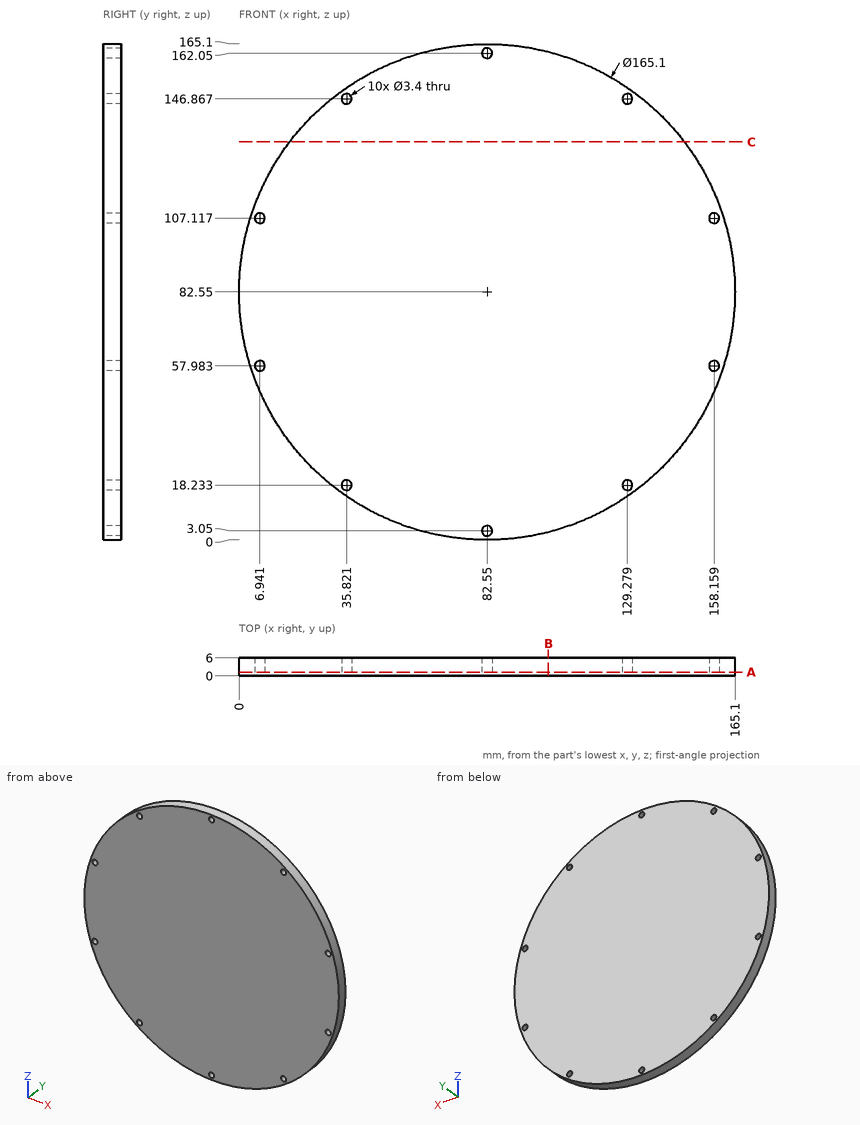
Design review of the part shown in the three views and the two pictorial views. Dimensions are in mm from the part's minimum x, y and z. Give positions to 0.01 mm unless a question says otherwise; leave off trailing zeros. Write each loop counter-clockwise with the first axis right and the second up, starting at its lowest first coordinate (ties: lowest second). Pieces come first, ordered by that corner, then holes.
(1) Add section A-A (y = 1.3). Give the number of separate pieces and of enclosed holes in the cut face, and give its area (3 significant figures).
Checked values:
separate pieces: 1
enclosed holes: 10
area: 21,300 mm2
(2) Add section C-C (z = 132.5). Give the boundary of the cut face in (x, y), and give its area (3 significant figures).
Checked values:
outline: (16.83, 0) - (148.27, 0) - (148.27, 6) - (16.83, 6) - close
area: 789 mm2
(3) Add section B-B (x = 103). Give the boundary of the cut face in (y, z), and give its area (3 significant figures).
Checked values:
outline: (0, 2.57) - (6, 2.57) - (6, 162.53) - (0, 162.53) - close
area: 960 mm2
(4) Wall thickness on line 1 along Z through (x, y) = (82.55, 3.95); line 2 along Z through (x, y) = (36, 2.05); line 3 along X through (y, z) = (5.35, 80.5): over which ranges is each line inside the solid? List them lowest first.
Checked values:
line 1: z = 0 to 1.35, 4.75 to 160.35, 163.75 to 165.1
line 2: z = 14.38 to 16.54, 19.92 to 145.18, 148.56 to 150.72
line 3: x = 0.03 to 165.07
(5) Clearance check with flat-ended pins moving along their axes: pin 1 Ø2.5 at (x, z) = (82.55, 3.05) entering from +Y; pin 2 Ø1.5 at (y, z) = (4, 129) entering from -X; pin 3 Ø1 at (y, z) = (0.5, 127) entering from +X; pin 4 Ø1.5 at (y, z) = (2, 70.5) entering from +X. State where each tip first meets the part, or that it passes through.
Checked values:
pin 1: passes through
pin 2: stops at x = 13.8
pin 3: stops at x = 152.43
pin 4: stops at x = 164.32
